from build123d import *

# Parameters (mm, degrees)
F0_W     = 600
F0_H     = 600
F1_DEPTH = 30
F2_W     = 50
F2_H     = 50
F4_W     = 60.5461252972
F4_H     = 54.9688454909


with BuildPart() as f1:
    # F0 (on Top) → F1 (new body)
    with BuildSketch(Plane.XY):
        with Locations((-0.9914571419, -3.804606373)):
            Rectangle(F0_W, F0_H)
    extrude(amount=F1_DEPTH)

    # F7: F6_1, F5 across plane


with BuildPart() as f5:
    # F2 (on Top) → F5 section 0
    with BuildSketch(Plane.XY):
        with Locations((-216.2354439497, -223.8953137973)):
            Rectangle(F2_W, F2_H)
    # F4 (on offset) → F5 section 1
    with BuildSketch(Plane.XY.offset(-770)):
        with Locations((-295.7183944933, -301.3201836275)):
            Rectangle(F4_W, F4_H)
    loft()


with BuildPart() as f6_1:
    # F6: instance of F5
    add(f5.part.mirror(Plane.YZ))


with BuildPart() as f1_1:
    add(f1.part)
    add(f6_1.part.mirror(Plane.XZ))
    add(f5.part.mirror(Plane.XZ))


    add(f5.part)  # F19 merges F5

    add(f6_1.part)  # F19 merges F6_1
    # F19: F18 across plane


with BuildPart() as f10:
    # F9 (on face) → F10 section 0
    with BuildSketch(Plane(origin=(-189.4755147525, 0, 18.2609827385), x_dir=(0, 1, 0), z_dir=(0.9953878919, 0, -0.0959319791))):
        Polygon((259.3299424331, -642.1780271339), (264.1481227465, -691.9133727984), (318.4746398428, -691.9133727984), (313.336995282, -642.1780271339), align=None)
    # F8 (on face) → F10 section 1
    with BuildSketch(Plane(origin=(189.4755147525, 0, 18.2609827385), x_dir=(0, -1, 0), z_dir=(-0.9953878919, 0, -0.0959319791))):
        Polygon((-313.336995282, -642.1780271339), (-318.4746398428, -691.9133727984), (-264.1481227465, -691.9133727984), (-259.3299424331, -642.1780271339), align=None)
    loft()


with BuildPart() as f11_1:
    # F11: instance of F10
    add(f10.part.mirror(Plane.XZ))


with BuildPart() as f14:
    # F13 (on face) → F14 section 0
    with BuildSketch(Plane(origin=(0, 197.0290144931, 19.175899266), x_dir=(1, 0, 0), z_dir=(0, -0.9952972799, -0.0968675625))):
        Polygon((-255.8530072263, -692.904708192), (-251.0853709275, -643.202091898), (-309.5907715802, -643.202091898), (-315.0359468324, -692.904708192), align=None)
    # F12 (on face) → F14 section 1
    with BuildSketch(Plane(origin=(0, -197.0290144931, 19.175899266), x_dir=(-1, 0, 0), z_dir=(0, 0.9952972799, -0.0968675625))):
        Polygon((251.0853709275, -643.202091898), (255.8530072263, -692.904708192), (315.0359468324, -692.904708192), (309.5907715802, -643.202091898), align=None)
    loft()


with BuildPart() as f15_1:
    # F15: instance of F14
    add(f14.part.mirror(Plane.YZ))


with BuildPart() as f18:
    # F17 (on face) → F18 section 0
    with BuildSketch(Plane(origin=(-189.4755147525, 0, 18.2609827385), x_dir=(0, 1, 0), z_dir=(0.9953878919, 0, -0.0959319791))):
        Polygon((254.0329583581, -68.080940268), (248.8953137973, -18.3455946035), (198.8953137973, -18.3455946035), (203.7134941108, -68.080940268), align=None)
    # F16 (on face) → F18 section 1
    with BuildSketch(Plane(origin=(189.4755147525, 0, 18.2609827385), x_dir=(0, -1, 0), z_dir=(-0.9953878919, 0, -0.0959319791))):
        Polygon((-198.8953137973, -18.3455946035), (-248.8953137973, -18.3455946035), (-254.0329583581, -68.080940268), (-204.1813530846, -72.9103833916), align=None)
    loft()


with BuildPart() as f1_2:
    add(f1_1.part)
    add(f18.part.mirror(Plane.XZ))



with BuildPart() as f22:
    # F21 (on face) → F22 section 0
    with BuildSketch(Plane(origin=(0, 197.0290144931, 19.175899266), x_dir=(1, 0, 0), z_dir=(0, -0.9952972799, -0.0968675625))):
        Polygon((-190.9130329513, -19.2665042431), (-241.2354439497, -19.2665042431), (-246.6847009277, -69.0063778227), (-196.0066540883, -69.0063778227), align=None)
    # F20 (on face) → F22 section 1
    with BuildSketch(Plane(origin=(0, -197.0290144931, 19.175899266), x_dir=(-1, 0, 0), z_dir=(0, 0.9952972799, -0.0968675625))):
        Polygon((241.2354439497, -19.2665042431), (190.9130329513, -19.2665042431), (196.0066540883, -69.0063778227), (246.6806192019, -68.9691205372), align=None)
    loft()


with BuildPart() as f1_3:
    add(f1_2.part)

    add(f10.part)  # F23 merges F10

    add(f11_1.part)  # F23 merges F11_1

    add(f14.part)  # F23 merges F14

    add(f15_1.part)  # F23 merges F15_1

    add(f18.part)  # F23 merges F18

    add(f22.part)  # F23 merges F22
    # F23: F22 across plane
    add(f22.part.mirror(Plane.YZ))


solid = f1_3.part
Check sheet for the modelled part. Datum: model origin and axes. Units: mm. A direction names the side the tool comes from. Round coordinates to 2 decimals unless told otherwise and drop trailing zeros.
(1) Draft check along X on faces 5 (the flat face through (299.009, -8, 15)), 6 (the flat face through (-5, 0, 30)), 7 (the flat face through (4, -291, -670.461)). Enter one of: pulls with the +X half, pulls with the -X half, needs draft (parallel to the pull), parting line crosses it, or undercut.
(2) Scan lines: probe 1 along Y at (x, z) = (-291, -585); probe 2 along Z at (x, y) = (170.5, -81.5); probe 3 along X at (y, z) = (224, -243.5). Record each from-to range of solid material in increasing order.
(3) Cross-section at A-A, the plane y = -65. State how many separate pieces and enclosed holes the cut face has, and give its area (3 significant figures).
(4) Go/stop test with flat-tipped pins: P1, Ø18, axis at x = 274, y = -90.5, coming from the -Z side; P2, Ø15, axis at y = -37, z = 13.5, coming from the +X side; P3, Ø15, axis at x = -78, z = 21, coming from the +Y side. Record where each tip stops, or that it passes through.
(5) Access from +Z, -Z, +X, -X, +Y, -Y to the whole of each face (thin tool, end or side, straight path). Record for faces 1 (the flat face through (-286, -4, -670.47)), 2 (the flat face through (-3, 3, 0)), 3 (the flat face through (-280, -4, -621.001)), 4 (the flat face through (-5, 296.195, 15)).
Check sheet entries:
1. face 5: pulls with the +X half
1. face 6: needs draft
1. face 7: undercut
2. probe 1: y = -309.61 to -255.83, 255.83 to 309.61
2. probe 2: z = 0 to 30
2. probe 3: x = -268.04 to -214.7, 214.7 to 268.04
3. separate pieces: 3
3. enclosed holes: 0
3. area: 28,800 mm2
4. P1: stops at z = -670.47
4. P2: stops at x = 299.01
4. P3: stops at y = 296.2
5. face 1: -Z, +X, -X
5. face 2: -Z
5. face 3: +X, -X
5. face 4: +Z, +X, -X, +Y
